Check sheet for the drawn part. Datum: minimum x, y, z corner. Units: mm. A direction names the side the tool comes from. Round coordinates to 2 decimals unless told otherwise and drop trailing zeros. Write each loop counter-clockwise with the first axis right and the second up, starting at its lowest first coordinate (ties: lowest second). Pieces come first, ordered by that corner, then holes. Notation, with made-up numbers: (53, -2.5) - (111, -2.5) arc R20 ccw to (111, 35.5) - close; hole circle Ø10 at (26.25, 62). An arc over 180 degrees is marked (long way). Answer as a JSON object with one key per item and string values. Group by question number.
Item 1: Release check for a two-part mould opening along X. For the marked faces 1, 2 and 3 record: pulls with the +X half, pulls with the -X half, needs draft (parallel to the pull), parting line crosses it, or undercut.
Item 2: Sectioned sample at D-D on x = 7. Record the boundary of the cut face in (y, z), plus the area to 3 significant figures.
Item 3: Gauge pin test, flat ends, axial feed: P1, Ø1, axis at y = 11.5, z = 3, coming from the +X side; P2, Ø1.5, axis at y = 30, z = 4.5, coming from the +X side; P3, Ø2, axis at x = 26.5, z = 2, coming from the -Y side. Record the tip position at first contact, or that the pin passes through.
Item 4: Thickness scan on line 1 (Y direction, x = 18.5, z = 0.2); line 2 (Y direction, x = 18.5, z = 7.25); line 3 (Z direction, x = 12, y = 6.5). Record the ranges inside material, lowest first.
Item 5: Sectioned sample at C-C on z = 5.25. Record the boundary of the cut face in (x, y), plus the area to 3 significant figures.
Item 6: Sectioned sample at A-A on y = 18.5. Record the boundary of the cut face in (x, z), plus the area to 3 significant figures.
Item 7: Set-up check for the marked faces 4, 5 and 6: record each of +Z, -Z, +X, -X, +Y, -Y from which the full face is reachable in a straight line by a thin tool's end or side.
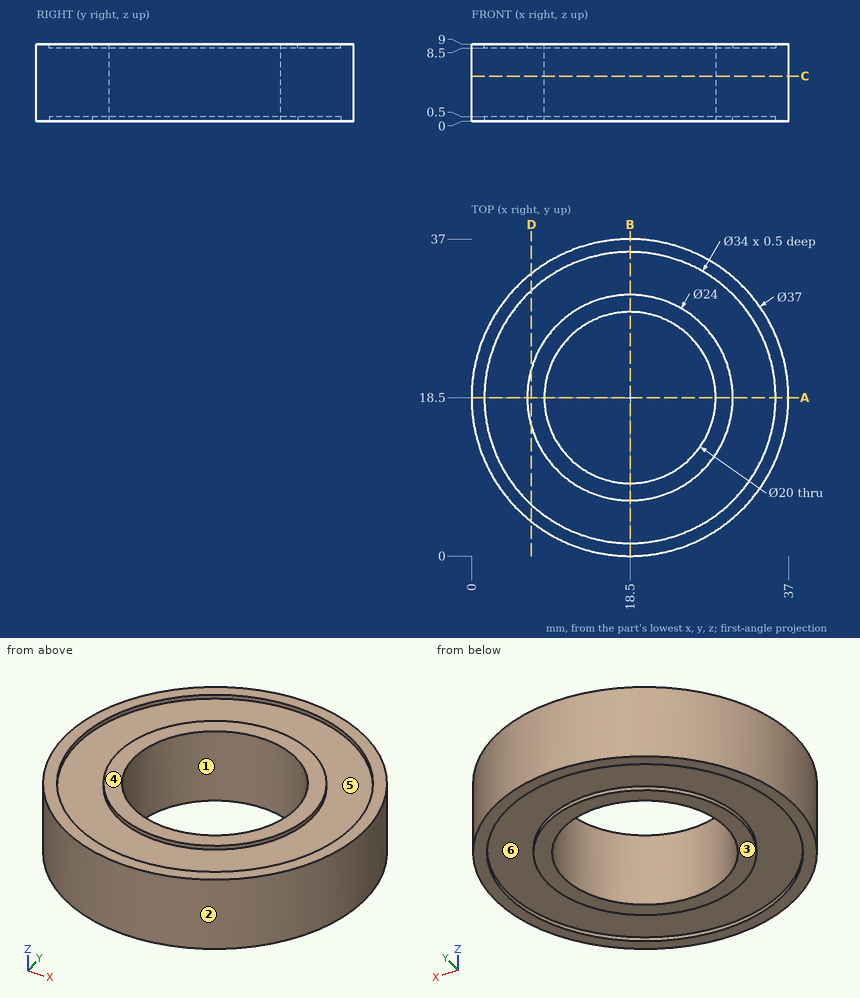
Completed:
{
 "1": {"face 1": "undercut", "face 2": "parting line crosses it", "face 3": "needs draft"},
 "2": {"outline": "(4.01, 0) - (5.98, 0) - (5.98, 0.5) - (15.07, 0.5) - (15.07, 0) - (21.93, 0) - (21.93, 0.5) - (31.02, 0.5) - (31.02, 0) - (32.99, 0) - (32.99, 9) - (31.02, 9) - (31.02, 8.5) - (21.93, 8.5) - (21.93, 9) - (15.07, 9) - (15.07, 8.5) - (5.98, 8.5) - (5.98, 9) - (4.01, 9) - close", "area": "243 mm²"},
 "3": {"P1": "x = 35.82", "P2": "x = 33.56", "P3": "y = 1.38"},
 "4": {"line 1": "0 to 1.5, 6.5 to 8.5, 28.5 to 30.5, 35.5 to 37", "line 2": "0 to 8.5, 28.5 to 37", "line 3": "0.5 to 8.5"},
 "5": {"outline": "circle Ø37 at (18.5, 18.5); hole circle Ø20 at (18.5, 18.5)", "area": "761 mm²"},
 "6": {"outline": "(0, 0) - (1.5, 0) - (1.5, 0.5) - (6.5, 0.5) - (6.5, 0) - (8.5, 0) - (8.5, 9) - (6.5, 9) - (6.5, 8.5) - (1.5, 8.5) - (1.5, 9) - (0, 9) - close; (28.5, 0) - (30.5, 0) - (30.5, 0.5) - (35.5, 0.5) - (35.5, 0) - (37, 0) - (37, 9) - (35.5, 9) - (35.5, 8.5) - (30.5, 8.5) - (30.5, 9) - (28.5, 9) - close", "area": "143 mm²"},
 "7": {"face 4": "+Z, +X, -X, +Y, -Y", "face 5": "+Z", "face 6": "-Z"}
}
